from build123d import *

# Parameters (mm, degrees)
F0_R        = 4
F0_R_2      = 2.85
F1_DEPTH    = 4
F2_DEPTH    = 6
F3_R        = 3.99999
F4_SIZE     = 0.5
F5_S5_R     = 4
F5_T6_DEPTH = 7


# Not quite as in the source:
# - a fillet or chamfer that OpenCascade refuses, or shapes differently, is made with other operations: its cross-section is extruded or revolved along the edge and cut away or added
# - a fillet or chamfer is up to 0.001 mm smaller than in the source, because OpenCascade refuses the exact size


with BuildPart() as f1:
    # F0 (on Top) → F1 (new body)
    with BuildSketch(Plane.XY):
        Circle(F0_R)
        Circle(F0_R_2, mode=Mode.SUBTRACT)
        Circle(F0_R_2)
    extrude(amount=F1_DEPTH)

    # F0 (on Top) → F2 (join)
    with BuildSketch(Plane.XY):
        Circle(F0_R_2)
    extrude(amount=-F2_DEPTH)

    # F3 (radius 4 in the source; OpenCascade refuses exactly that, so slightly less here)
    f3_edges = [f1.edges().sort_by_distance(p)[0] for p in [
        (-4, 0, 4),
    ]]
    fillet(f3_edges, radius=F3_R)

    # F4
    f4_edges = [f1.edges().sort_by_distance(p)[0] for p in [
        (-2.85, 0, -6),
    ]]
    chamfer(f4_edges, length=F4_SIZE)

    # F5: chamfer of 1.2 x 1.0069195574 on 1 edges, made by hand


with BuildPart() as f5_tool2:
    # F5_s3 → F5_t4 (revolve)
    with BuildSketch(Plane.XZ):
        Polygon((2.85, -1.0069195574), (4.05, 0), (2.85, 0), align=None)
    revolve(axis=Axis((0, 0, 0), (0, 0, 1)))

    # F5_s5 → F5_t6 (intersect, symmetric)
    with BuildSketch(Plane.XY.offset(-0.5)):
        Circle(F5_S5_R)
    extrude(amount=F5_T6_DEPTH, both=True, mode=Mode.INTERSECT)


with BuildPart() as f1_1:
    add(f1.part)

    # F5_t1: union F5_tool2
    add(f5_tool2.part)


solid = f1_1.part
CAD build for the part. Positions are in the model's coordinates, mm. A direction names the side the tool comes from. Round coordinates to 2 decimals unless told otherwise and drop trailing zeros. Write each loop counter-clockwise with the first axis right and the second up, starting at its lowest first coordinate (ties: lowest second). Pieces come first, ordered by that corner, then holes.
(1) Slice it at A-A, the plane z = -4.25. Write the cut outline in (x, y), and give its area (3 significant figures).
(2) 3-axis set-ups, long thin cutter, end or side, ignore diameter. For faces 1 (the face through (-2.262, -1.734, -3.222)), 2 (the face through (0, 0, -6)): which of +Z, -Z, +X, -X, +Y, -Y reach the whole face in a straight line?
(3) Probe line 1 along X through (y, z) = (-3.25, 0.5); line 2 along Z through (x, y) = (-2.25, 3); line 3 along X through (y, z) = (-2.5, -2). List the from-to ranges inside material, lowest first.
(4) Drop flat-ended pins along their axis: P1, Ø1.5, axis at x = 1, z = -4, coming from the -Y side; P2, Ø2, axis at y = 0, z = 2, coming from the -X side; P3, Ø1.5, axis at x = 2.5, z = -4, coming from the +Y side. Give the stop position or say it passes through.
From the geometry:
1. outline: circle Ø5.7 at (0, 0)
1. area: 25.5 mm2
2. face 1: -Z
2. face 2: -Z, +X, -X, +Y, -Y
3. line 1: x = -2.28 to 2.28
3. line 2: z = -0.25 to 1.39
3. line 3: x = -1.37 to 1.37
4. P1: stops at y = -2.84
4. P2: stops at x = -3.87
4. P3: stops at y = 2.25
